Print and shaded views of the part. All mm, measured from the part's lowest x, y and z. A direction names the side the tool comes from. Round coordinates to 2 decimals unless told otherwise and drop trailing zeros. Write each loop counter-clockwise with the first axis right and the second up, starting at its lowest first coordinate (ties: lowest second). Pieces come first, ordered by that corner, then holes. Notation, with made-up numbers: (15.25, -3) - (32.25, -3) arc R19 cw to (32.25, 12) - close; hole circle Ø8 at (-19.5, 88.25). An arc over 180 degrees is marked (long way). Put each result on its own line as item: value. Start each with the question number.
Item 1: 3-axis set-ups, long thin cutter, end or side, ignore diameter. For the marked faces 4 and 5: which of +Z, -Z, +X, -X, +Y, -Y reach the whole face in a straight line?
Item 2: Cut at A-A (y = 3.25). Give the cut face in (x, z).
Item 3: Pin check, flat tip, straight feed: pin 1 Ø1.5 at (y, z) = (7.5, 2) entering from -X. Stop position of the tip, or through.
Item 4: Cut at C-C (z = 2.35). Give the cut face in (x, y) (1 decimal), and give its area (3 significant figures).
Item 5: Drill centre lines: line 1 (X direction, y = 3.5, z = 2.4); line 2 (X direction, y = 11.25, z = 1.6) (1 decimal); line 3 (Y direction, x = 18.5, z = 2) (1 decimal). Where is each one in solid material? Low to high. Write a range as from..to.
Item 6: Mould opens along X. For the marked faces 1, 2 and 3 say: released by +X, released by -X, zero draft, split by the parting line, or undercut.
Item 7: Cut at B-B (x = 20). Give the cut face in (y, z).
Item 8: Cut at D-D (x = 27). Give the cut face in (y, z).
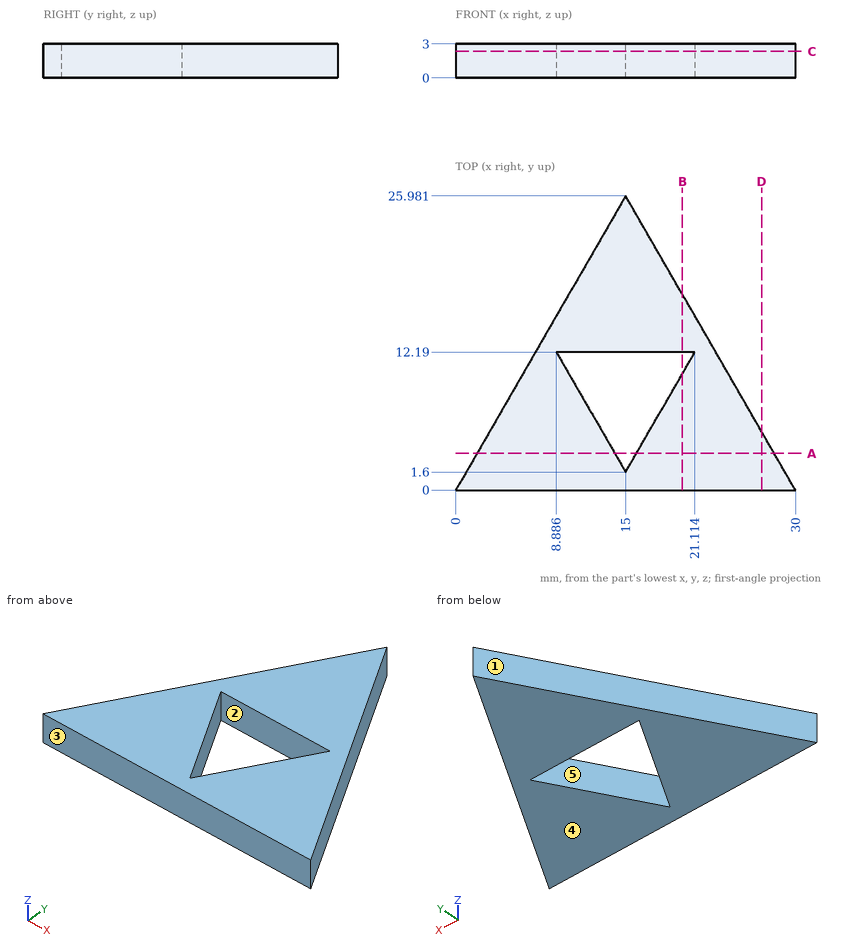
Output values:
1. face 4: -Z, +X, -X, +Y, -Y
1. face 5: +Z, -Z
2. outline: (1.88, 0) - (14.05, 0) - (14.05, 3) - (1.88, 3) - close; (15.95, 0) - (28.12, 0) - (28.12, 3) - (15.95, 3) - close
3. pin 1: x = 3.9
4. outline: (0, 0) - (30, 0) - (15, 26) - close; hole (8.9, 12.2) - (15, 1.6) - (21.1, 12.2) - close
4. area: 325 mm2
5. line 1: 2.02..13.9, 16.1..27.98
5. line 2: 6.5..9.4, 20.6..23.5
5. line 3: 0..7.7, 12.2..19.9
6. face 1: released by -X
6. face 2: undercut
6. face 3: zero draft
7. outline: (0, 0) - (10.26, 0) - (10.26, 3) - (0, 3) - close; (12.19, 0) - (17.32, 0) - (17.32, 3) - (12.19, 3) - close
8. outline: (0, 0) - (5.2, 0) - (5.2, 3) - (0, 3) - close
